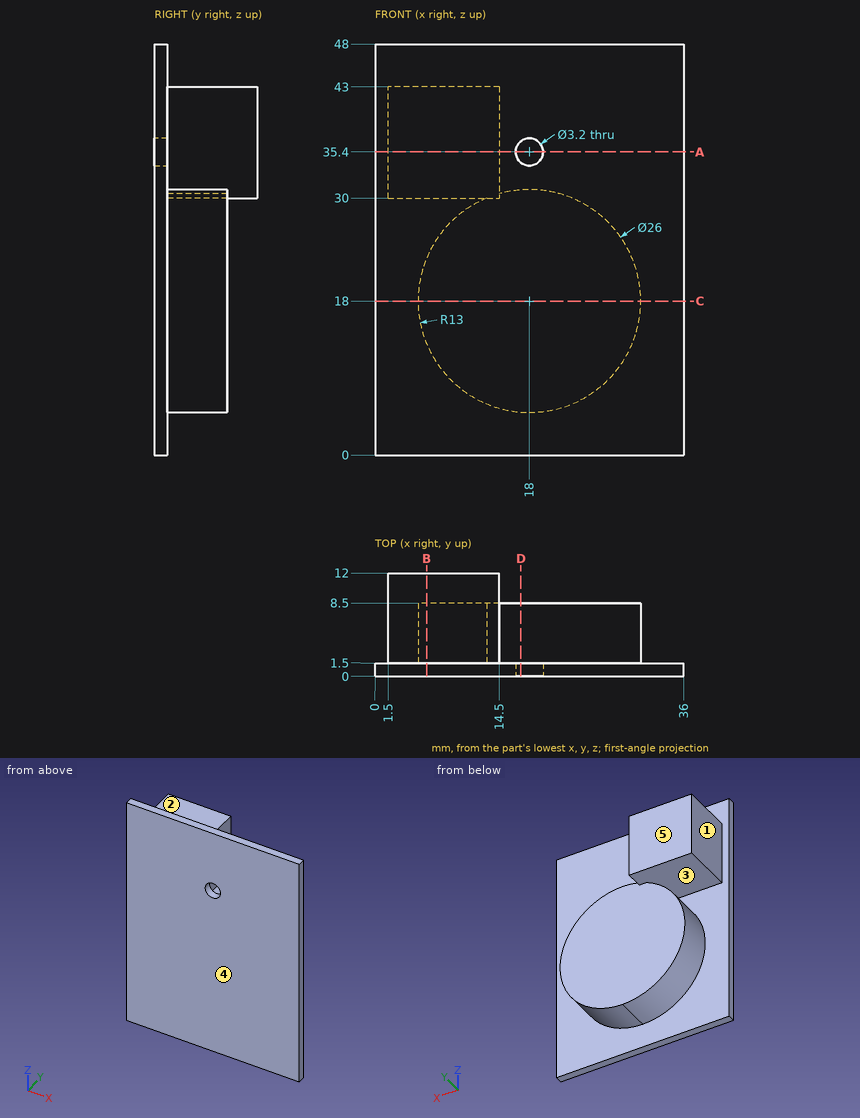
Check sheet for the drawn part. Datum: minimum x, y, z corner. Units: mm. A direction names the side the tool comes from. Give positions to 0.01 mm unless a question says otherwise; leave off trailing zeros. Order: outer loops, then holes, each group sorted by start corner. A loop starts at its lowest first (then second) coordinate and runs counter-clockwise, first axis right, second up. Notation, with made-up numbers: (82, -27) -> (127, -27) arc R17 ccw to (127, -19) -> close; hole circle Ø10 at (68.25, 17.25). An arc over 180 degrees is marked (long way). One line per item, written item: value.
(1) Gauge pin test, flat ends, axial feed: pin 1 (10 mm diameter, centred on x = 25.5, z = 9, fed in from -Y); pin 2 (3 mm diameter, centred on y = 9, z = 38.5, fed in from -X); pin 3 (1.5 mm diameter, centred on x = 13, y = 4.5, fed in from +Z); pin 4 (5 mm diameter, centred on x = 7.5, y = 6.5, fed in from -Z). Record the tip position at first contact, or that the pin passes through.
Final values:
pin 1: y = 0
pin 2: x = 1.5
pin 3: z = 43
pin 4: z = 7.75
(2) Sectioned sample at C-C on z = 18. Record the cut outline in (x, y).
Final values:
outline: (0, 0) -> (36, 0) -> (36, 1.5) -> (31, 1.5) -> (31, 8.5) -> (5, 8.5) -> (5, 1.5) -> (0, 1.5) -> close
(3) Sectioned sample at A-A on z = 35.4. Record the cut outline in (x, y), then the cut area to 3 significant figures.
Final values:
outline: (0, 0) -> (16.4, 0) -> (16.4, 1.5) -> (14.5, 1.5) -> (14.5, 12) -> (1.5, 12) -> (1.5, 1.5) -> (0, 1.5) -> close; (19.6, 0) -> (36, 0) -> (36, 1.5) -> (19.6, 1.5) -> close
area: 186 mm^2
(4) Scan lines: line 1 along Z through (x, y) = (18, 1.1); line 2 along X through (y, z) = (0.9, 35.4); line 3 along Y through (x, z) = (28.5, 39.5). Record each from-to range of solid material in increasing order. Write a range as [from, to].
Final values:
line 1: [0, 33.8], [37, 48]
line 2: [0, 16.4], [19.6, 36]
line 3: [0, 1.5]
(5) Sectioned sample at D-D on x = 17. Record the cut outline in (y, z), then the cut area to 3 significant figures.
Final values:
outline: (0, 0) -> (1.5, 0) -> (1.5, 5.04) -> (8.5, 5.04) -> (8.5, 30.96) -> (1.5, 30.96) -> (1.5, 34.15) -> (0, 34.15) -> close; (0, 36.65) -> (1.5, 36.65) -> (1.5, 48) -> (0, 48) -> close
area: 250 mm^2
(6) Tool access check on the marked faces 1, 2, 3, 4 and 5. Record the directions out of +Z, -Z, +X, -X, +Y, -Y that give a thin tool (end or side, any length) a straight path to the whole face; none if there is none.
Final values:
face 1: +Z, -Z, -X, +Y
face 2: +Z, +X, -X, +Y
face 3: -X, +Y
face 4: +Z, -Z, +X, -X, -Y
face 5: +Z, -Z, +X, -X, +Y
(7) Sectioned sample at B-B on x = 6. Record the cut outline in (y, z).
Final values:
outline: (0, 0) -> (1.5, 0) -> (1.5, 13) -> (8.5, 13) -> (8.5, 23) -> (1.5, 23) -> (1.5, 30) -> (12, 30) -> (12, 43) -> (1.5, 43) -> (1.5, 48) -> (0, 48) -> close
